Read the model definition and answer for the solid it produces. Units are mm, in the model's axes. Face numbers are marked on the shaded views. A direction names the side the tool comes from. Give positions to 0.01 mm unless a question says otherwise; leave off trailing zeros. Loops run counter-clockwise (first coordinate to the right, second up) from the corner with the lowest first, then second, coordinate; pieces in that order, holes last. Notation, with made-up numbers: (-37.5, 50) - (-32.5, 50) arc R19 cw to (-32.5, 63) - close; hole circle Ø10 at (-11.5, 28). An arc over 180 degrees is marked (long way). Write item = value, one per line.
```python
from build123d import *
from build123d.topology import SkipClean

# Parameters (mm, degrees)
SKETCH1_R           = 0.75
BOSS_EXTRUDE1_DEPTH = 24
BOSS_EXTRUDE2_START = 7
SKETCH2_R           = 8
SKETCH2_R_2         = 2.65
BOSS_EXTRUDE2_DEPTH = 7
SKETCH4_W           = 5
SKETCH4_H           = 11
CUT_EXTRUDE1_DEPTH  = 39.600518131
SKETCH5_R           = 1.75
CUT_EXTRUDE2_DEPTH  = 32.957002363
SKETCH6_R           = 1.75
CUT_EXTRUDE3_DEPTH  = 29.517538579


with BuildPart() as part:
    # Sketch1 → Boss-Extrude1 (new body)
    with BuildSketch(Plane.XY):
        with BuildLine():
            Line((-12.5, 0), (12.5, 0))
            Line((12.5, 0), (12.5, 6))
            Line((12.5, 6), (6.302543671, 13.927265294))
            ThreePointArc((6.302543671, 13.927265294), (0, 17), (-6.302543671, 13.927265294))
            Line((-6.302543671, 13.927265294), (-12.5, 6))
            Line((-12.5, 6), (-12.5, 0))
        make_face()
        with Locations((0, 9)):
            Circle(SKETCH1_R, mode=Mode.SUBTRACT)
    extrude(amount=BOSS_EXTRUDE1_DEPTH)

    # Sketch2 → Boss-Extrude2 (add)
    with SkipClean():  # the faces are left unmerged after this step: merging them gives an invalid solid
        with BuildSketch(Plane(origin=(0, 0, 0), x_dir=(-1, 0, 0), z_dir=(0, 0, -1)).offset(BOSS_EXTRUDE2_START)):
            with Locations((0, 9)):
                Circle(SKETCH2_R)
            with Locations((0, 9)):
                Circle(SKETCH2_R_2, mode=Mode.SUBTRACT)
        extrude(amount=-BOSS_EXTRUDE2_DEPTH)

    # Sketch4 → Cut-Extrude1 (cut, through all)
    with BuildSketch(Plane(origin=(12.5, 0, 0), x_dir=(0, 0, -1), z_dir=(1, 0, 0))):
        with Locations((-12, 11.5)):
            Rectangle(SKETCH4_W, SKETCH4_H)
    extrude(amount=-CUT_EXTRUDE1_DEPTH, mode=Mode.SUBTRACT)

    # Sketch5 → Cut-Extrude2 (cut, through all)
    with SkipClean():  # the faces are left unmerged after this step: merging them gives an invalid solid
        with BuildSketch(Plane.XZ):
            with Locations(Location((0, 19.25, 0), (0, 0, 270))):
                Circle(SKETCH5_R)
        extrude(amount=-CUT_EXTRUDE2_DEPTH, mode=Mode.SUBTRACT)

    # Sketch6 → Cut-Extrude3 (cut, through all)
    with SkipClean():  # the faces are left unmerged after this step: merging them gives an invalid solid
        with BuildSketch(Plane(origin=(0, 9, 0), x_dir=(-1, 0, 0), z_dir=(0, -1, 0))):
            with Locations(Location((0, 2.25, 0), (0, 0, 90))):
                Circle(SKETCH6_R)
        extrude(amount=-CUT_EXTRUDE3_DEPTH, mode=Mode.SUBTRACT)


solid = part.part
```
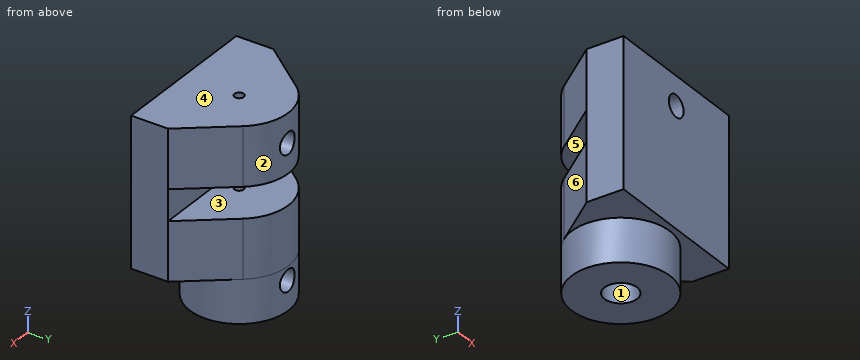
1) Find the intervals of material crossed by probe 1 along Y at (x, z) = (0, 4); probe 2 along Z at (x, y) = (6, 14.25); probe 3 along X at (y, z) = (9, 15.9), in increasing order.
Output:
probe_1 = 0 to 8.25, 9.75 to 17
probe_2 = -7 to 9.5, 14.5 to 24
probe_3 = -10.15 to -0.75, 0.75 to 10.15
2) A tool of negligible diameter and unlimited length cuts with its end or side. For the marked faces 1, 2 and 3, from which of +Z, -Z, +X, -X, +Y, -Y can it reach the whole face along a straight path? Write none if from no direction.
Output:
face_1 = -Z
face_2 = +Z, -Z, +Y
face_3 = +X, -X, +Y
3) Each of these flat-tipped pins is pushed along its axis until it touches: P1, Ø2, axis at x = 0, z = 19.25, coming from the -Y side; P2, Ø2.5, axis at x = -4.5, z = 12, coming from the +Y side; P3, Ø3, axis at x = 9, z = 4, coming from the +Y side; P4, Ø1.5, axis at x = 1, z = 17, coming from the +Y side. Where does it stop, or does it pass through?
Output:
P1 = through
P2 = 6
P3 = 12.4
P4 = 17
4) The mould has two halves that part along Z. Classify the marked faces 4, 5 and 6: pulls with the +Z half, pulls with the -Z half, needs draft (parallel to the pull), parting line crosses it, or undercut.
Output:
face_4 = pulls with the +Z half
face_5 = undercut
face_6 = needs draft
5) A cutting plane is placed at C-C on y = 9. Determine the outline of the cut face in (x, z), then the cut area to 3 significant figures.
Output:
outline = (-10.15, 0) - (-8, 0) - (-8, -7) - (-2.65, -7) - (-2.65, 0) - (-0.75, 0) - (-0.75, 9.5) - (-10.15, 9.5) - close; (-10.15, 14.5) - (-0.75, 14.5) - (-0.75, 17.67) arc R1.75 cw to (-0.75, 20.83) - (-0.75, 24) - (-10.15, 24) - close; (0.75, 0) - (2.65, 0) - (2.65, -7) - (8, -7) - (8, 0) - (10.15, 0) - (10.15, 9.5) - (0.75, 9.5) - close; (0.75, 14.5) - (10.15, 14.5) - (10.15, 24) - (0.75, 24) - (0.75, 20.83) arc R1.75 cw to (0.75, 17.67) - close
area = 428 mm²
6) A cutting plane is placed at B-B on x = 0. Give the number of separate pieces and of enclosed holes in the cut face, then the cut area to 3 significant figures.
Output:
separate_pieces = 6
enclosed_holes = 0
area = 326 mm²
7) A cutting plane is placed at A-A on z = 1. Determine the outline of the cut face in (x, y).
Output:
outline = (-12.5, 0) - (12.5, 0) - (12.5, 6) - (6.3, 13.93) arc R8 ccw to (-6.3, 13.93) - (-12.5, 6) - close; hole circle Ø1.5 at (0, 9)
8) A cutting plane is placed at D-D on y = 3.75. Determine the outline of the cut face in (x, z), then the cut area to 3 significant figures.
Output:
outline = (-12.5, 0) - (-6.04, 0) - (-6.04, -7) - (6.04, -7) - (6.04, 0) - (12.5, 0) - (12.5, 24) - (-12.5, 24) - close; hole circle Ø3.5 at (0, 19.25)
area = 675 mm²
